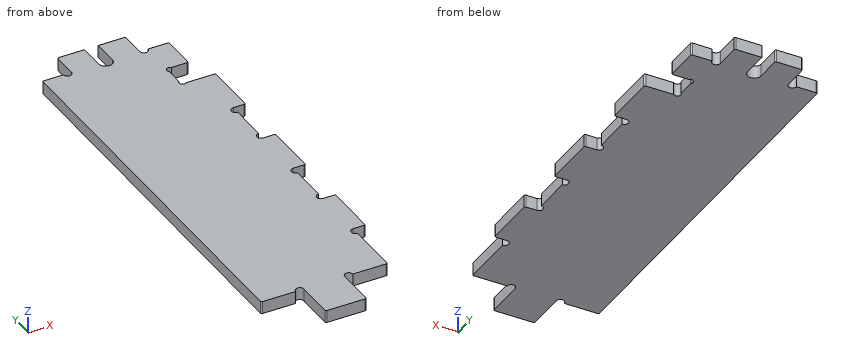
from build123d import *

# Parameters (mm, degrees)
BOSS_EXTRUDE1_DEPTH = 4.6
CUT_EXTRUDE1_DEPTH  = 164.683291756
SKETCH8_W           = 8
SKETCH8_H           = 10
CUT_EXTRUDE4_DEPTH  = 10
SKETCH9_R           = 1.25
CUT_EXTRUDE5_DEPTH  = 10
FILLET1_R           = 0.5


with BuildPart() as part:
    # Sketch1 → Boss-Extrude1 (new body)
    with BuildSketch(Plane.XY):
        Polygon((10.7, 146), (10.7, 155.5), (20.7, 155.5), (20.7, 146), (25.7, 146), (25.7, 155.5), (35.7, 155.5), (35.7, 146), (46.4, 146), (46.4, 123), (50.9, 123), (50.9, 103), (46.4, 103), (46.4, 83), (50.9, 83), (50.9, 63), (46.4, 63), (46.4, 43), (50.9, 43), (50.9, 23), (46.4, 23), (46.4, 0), (30.7, 0), (30.7, -14.5), (15.7, -14.5), (15.7, 0), (0, 0), (0, 146), align=None)
    extrude(amount=BOSS_EXTRUDE1_DEPTH)

    # Sketch2 → Cut-Extrude1 (cut, through all)
    with BuildSketch(Plane.XY.offset(4.6)):
        with BuildLine():
            Line((15.7, 0), (15.7, -5))
            ThreePointArc((15.7, -5), (14.2, -6.5), (12.7, -5))
            Line((12.7, -5), (12.7, 0))
            ThreePointArc((12.7, 0), (14.2, 1.5), (15.7, 0))
        make_face()
        with BuildLine():
            Line((30.7, 0), (30.7, -5))
            ThreePointArc((30.7, -5), (32.2, -6.5), (33.7, -5))
            Line((33.7, -5), (33.7, 0))
            ThreePointArc((33.7, 0), (32.2, 1.5), (30.7, 0))
        make_face()
        with BuildLine():
            Line((46.4, 23), (50.9, 23))
            ThreePointArc((50.9, 23), (52.4, 21.5), (50.9, 20))
            Line((50.9, 20), (46.4, 20))
            ThreePointArc((46.4, 20), (44.9, 21.5), (46.4, 23))
        make_face()
        with BuildLine():
            Line((46.4, 63), (50.9, 63))
            ThreePointArc((50.9, 63), (52.4, 61.5), (50.9, 60))
            Line((50.9, 60), (46.4, 60))
            ThreePointArc((46.4, 60), (44.9, 61.5), (46.4, 63))
        make_face()
        with BuildLine():
            Line((46.4, 103), (50.9, 103))
            ThreePointArc((50.9, 103), (52.4, 101.5), (50.9, 100))
            Line((50.9, 100), (46.4, 100))
            ThreePointArc((46.4, 100), (44.9, 101.5), (46.4, 103))
        make_face()
        with BuildLine():
            Line((46.4, 43), (50.9, 43))
            ThreePointArc((50.9, 43), (52.4, 44.5), (50.9, 46))
            Line((50.9, 46), (46.4, 46))
            ThreePointArc((46.4, 46), (44.9, 44.5), (46.4, 43))
        make_face()
        with BuildLine():
            Line((46.4, 83), (50.9, 83))
            ThreePointArc((50.9, 83), (52.4, 84.5), (50.9, 86))
            Line((50.9, 86), (46.4, 86))
            ThreePointArc((46.4, 86), (44.9, 84.5), (46.4, 83))
        make_face()
        with BuildLine():
            Line((35.7, 146), (35.7, 155.5))
            ThreePointArc((35.7, 155.5), (37.2, 157), (38.7, 155.5))
            Line((38.7, 155.5), (38.7, 146))
            ThreePointArc((38.7, 146), (37.2, 144.5), (35.7, 146))
        make_face()
        with BuildLine():
            Line((25.7, 146), (25.7, 155.5))
            ThreePointArc((25.7, 155.5), (23.2, 158), (20.7, 155.5))
            Line((20.7, 155.5), (20.7, 146))
            ThreePointArc((20.7, 146), (23.2, 143.5), (25.7, 146))
        make_face()
        with BuildLine():
            Line((10.7, 146), (10.7, 155.5))
            ThreePointArc((10.7, 155.5), (9.2, 157), (7.7, 155.5))
            Line((7.7, 155.5), (7.7, 146))
            ThreePointArc((7.7, 146), (9.2, 144.5), (10.7, 146))
        make_face()
    extrude(amount=-CUT_EXTRUDE1_DEPTH, mode=Mode.SUBTRACT)

    # Sketch8 → Cut-Extrude4 (cut)
    with BuildSketch(Plane(origin=(0, 0, 0), x_dir=(-1, 0, 0), z_dir=(0, 0, -1))):
        with Locations((-42.4, 128)):
            Rectangle(SKETCH8_W, SKETCH8_H)
    extrude(amount=-CUT_EXTRUDE4_DEPTH, mode=Mode.SUBTRACT)

    # Sketch9 → Cut-Extrude5 (cut)
    with BuildSketch(Plane(origin=(0, 0, 0), x_dir=(-1, 0, 0), z_dir=(0, 0, -1))):
        with Locations((-39.28, 132.112250035)):
            Circle(SKETCH9_R)
        with Locations((-39.28, 123.887749965)):
            Circle(SKETCH9_R)
    extrude(amount=-CUT_EXTRUDE5_DEPTH, mode=Mode.SUBTRACT)

    # Fillet1
    fillet1_edges = [part.edges().sort_by_distance(p)[0] for p in [
        (46.4, 133, 2.3),
        (0, 146, 2.3),
        (10.7, 155.5, 2.3),
        (20.7, 155.5, 2.3),
        (35.7, 155.5, 2.3),
        (46.4, 146, 2.3),
        (50.9, 123, 2.3),
        (50.9, 103, 2.3),
        (50.9, 83, 2.3),
        (50.9, 63, 2.3),
        (50.9, 43, 2.3),
        (50.9, 23, 2.3),
        (46.4, 0, 2.3),
        (30.7, -14.5, 2.3),
        (15.7, -14.5, 2.3),
        (0, 0, 2.3),
    ]]
    fillet(fillet1_edges, radius=FILLET1_R)


solid = part.part
Model file for the job. Use its own axes, mm. Coordinates: 2 decimals unless noted, no trailing zeros. Loops run counter-clockwise (first coordinate to the right, second up) from the corner with the lowest first, then second, coordinate; pieces in that order, holes last. Notation, with made-up numbers: (56.5, 38) -> (102.5, 38) arc R17 cw to (102.5, 63) -> close; hole circle Ø1 at (-1.5, 59.25). An arc over 180 degrees is marked (long way). Use one line per item in the form item = value. Start each with the question number.
(1) Cut at A-A on x = 43. Give the cut face in (y, z), and give its area (3 significant figures).
(2) Probe probe 1 along Y at (x, z) = (9, 2.3); probe 2 along X at (y, z) = (56, 0.6); probe 3 along X at (y, z) = (132, 3.55). List the from-to ranges inside material, lowest first. Write a range as from..to.
(3) Cut at C-C on x = 9.2. Give the cut face in (y, z).
(4) Flat gauge pins, fed straight in: pin 1 (2.5 mm diameter, centred on y = 150, z = 1.5, fed in from +X); pin 2 (1.4 mm diameter, centred on x = 4.5, z = 2.5, fed in from -Y); pin 3 (2 mm diameter, centred on x = 47.5, z = 2, fed in from +Y). Where does each tip first touch, or does it go through?
(5) Cut at B-B on y = 44.5. Give the cut face in (x, z).
Values:
q1.outline = (0, 0) -> (123, 0) -> (123, 4.6) -> (0, 4.6) -> close; (133, 0) -> (146, 0) -> (146, 4.6) -> (133, 4.6) -> close
q1.area = 626 mm2
q2.probe_1 = 0..144.51
q2.probe_2 = 0..46.4
q2.probe_3 = 0..38.04
q3.outline = (0, 0) -> (144.5, 0) -> (144.5, 4.6) -> (0, 4.6) -> close
q4.pin_1 = 35.7
q4.pin_2 = 0
q4.pin_3 = 123
q5.outline = (0, 0) -> (44.9, 0) -> (44.9, 4.6) -> (0, 4.6) -> close
